Autodesk Inventor part; units mm, degrees
ref_plane "YZ Plane" through (0, 0, 0) normal (1, 0, 0) x (0, 1, 0)
ref_plane "XZ Plane" through (0, 0, 0) normal (0, 1, 0) x (-1, 0, 0)
ref_plane "XY Plane" through (0, 0, 0) normal (0, 0, 1) x (1, 0, 0)
sketch "Sketch1" plane through (0, 0, 0) normal (0, 0, 1) x (1, 0, 0)
  circle A0 centre (0, 0) radius 2.5
  dimension "d0" = 5
extrude "Extrusion1" add sketch "Sketch1" along normal blind 50
sketch "Sketch2" plane through (0, 0, 50) normal (0, 0, 1) x (1, 0, 0)
  circle A0 centre (0, 0) radius 3.5
  dimension "d3" = 7
extrude "Extrusion2" add sketch "Sketch2" along normal blind 20
sketch "Sketch3" plane through (0, 0, 70) normal (0, 0, 1) x (1, 0, 0)
  point P0 (0, 0)
  point P1 (0, 0)
hole "Hole1" at (0, 0, 70) direction (0, 0, -1) diameter 5.2 depth 15
equation "\"fitTol\" = 0.2"
properties part number "RCPlaneConnectorTest2"
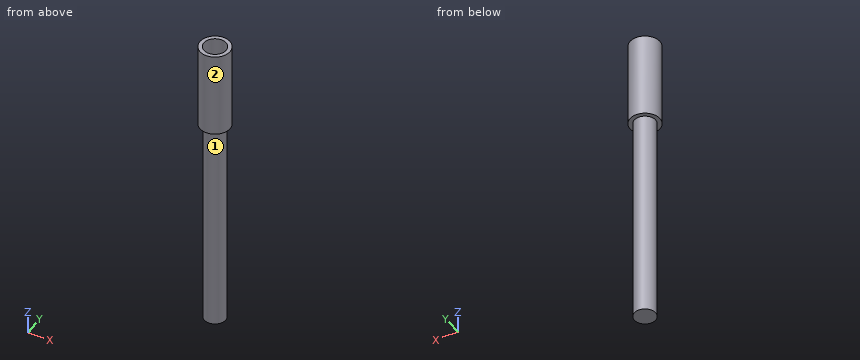
The listing builds one solid part. Answer for the finished solid, in the listing's coordinates (mm). Face numbers are marked on the shaded views. A direction names the side the tool comes from. Coordinates: 2 decimals unless noted, no trailing zeros. Loops run counter-clockwise (first coordinate to the right, second up) from the corner with the lowest first, then second, coordinate; pieces in that order, holes last.
1) Find the intervals of material crossed by L1, parallel to Y at x = 0, z = 62.75; L2, parallel to Z at x = 1.5, y = -0.5; L3, parallel to Z at x = -2, y = -2.25, in increasing order.
2) Find section C-C on z = 7. Write down the section's boundary in (x, y).
3) Find section A-A on y = 0. Write down the section's boundary in (x, z).
4) A tool of negligible diameter and unlimited length cuts with its end or side. For the marked faces 1 and 2, from which of +Z, -Z, +X, -X, +Y, -Y can it reach the whole face along a straight path? Write none if from no direction.
5) Flat-ended cylindrical pins translate along their axes: pin 1 Ø4 at (y, z) = (1.5, 35.5) entering from -X; pin 2 Ø2 at (x, z) = (-1.5, 9.5) entering from -Y; pin 3 Ø1.5 at (x, z) = (-2, 27.5) entering from +Y. Find the tip coordinate at first contact, or state that the pin passes through.
Values:
1. L1: y = -3.5 to -2.6, 2.6 to 3.5
1. L2: z = 0 to 55
1. L3: z = 50 to 70
2. outline: circle Ø5 at (0, 0)
3. outline: (-3.5, 50) - (-2.5, 50) - (-2.5, 0) - (2.5, 0) - (2.5, 50) - (3.5, 50) - (3.5, 70) - (2.6, 70) - (2.6, 55) - (-2.6, 55) - (-2.6, 70) - (-3.5, 70) - close
4. face 1: -Z
4. face 2: +Z, -Z
5. pin 1: stops at x = -2.5
5. pin 2: stops at y = -2.45
5. pin 3: stops at y = 2.17
